from build123d import *

# Parameters (mm, degrees)
SKETCH079_W     = 100
SKETCH079_H     = 40
PAD064_DEPTH    = 5
SKETCH080_W     = 5
SKETCH080_H     = 40
PAD065_DEPTH    = 15
SKETCH081_R     = 2.7
POCKET019_DEPTH = 100.001
SKETCH082_R     = 2.7
POCKET020_DEPTH = 5
SKETCH089_W     = 90
SKETCH089_H     = 5
PAD072_DEPTH    = 15


with BuildPart() as part:
    # Sketch079 → Pad064 (new body)
    with BuildSketch(Plane.XY):
        with Locations((50, 20)):
            Rectangle(SKETCH079_W, SKETCH079_H)
    extrude(amount=PAD064_DEPTH)

    # Sketch080 (on Face6 of Pad064) → Pad065 (join)
    with BuildSketch(Plane.XY.offset(5)):
        with Locations((2.5, 20)):
            Rectangle(SKETCH080_W, SKETCH080_H)
        with Locations((97.5, 20)):
            Rectangle(SKETCH080_W, SKETCH080_H)
    extrude(amount=PAD065_DEPTH)

    # Sketch081 (on Face5 of Pad065) → Pocket019 (cut, through all)
    with BuildSketch(Plane(origin=(0, 0, 0), x_dir=(0, -1, 0), z_dir=(-1, 0, 0))):
        with Locations((-30, 10)):
            Circle(SKETCH081_R)
        with Locations((-10, 10)):
            Circle(SKETCH081_R)
    extrude(amount=-POCKET019_DEPTH, mode=Mode.SUBTRACT)

    # Sketch082 (on Face8 of Pocket019) → Pocket020 (cut)
    with BuildSketch(Plane.XY.offset(5)):
        with Locations((14, 30)):
            Circle(SKETCH082_R)
        with Locations((14, 10)):
            Circle(SKETCH082_R)
        with Locations((86, 30)):
            Circle(SKETCH082_R)
        with Locations((86, 10)):
            Circle(SKETCH082_R)
        with Locations((50, 30)):
            Circle(SKETCH082_R)
        with Locations((50, 10)):
            Circle(SKETCH082_R)
    extrude(amount=-POCKET020_DEPTH, mode=Mode.SUBTRACT)

    # Sketch089 (on Face8 of Pocket020) → Pad072 (join)
    with BuildSketch(Plane.XY.offset(5)):
        with Locations((50, 37.5)):
            Rectangle(SKETCH089_W, SKETCH089_H)
        with Locations((50, 2.5)):
            Rectangle(SKETCH089_W, SKETCH089_H)
    extrude(amount=PAD072_DEPTH)


solid = part.part
Check sheet for the modelled part. Datum: model origin and axes. Units: mm. A direction names the side the tool comes from. Give positions to 0.01 mm unless a question says otherwise; leave off trailing zeros. Order: outer loops, then holes, each group sorted by start corner. A loop starts at its lowest first (then second) coordinate and runs counter-clockwise, first axis right, second up. Notation, with made-up numbers: M -39.75,-4 L 18.25,-4 A20 cw 18.25,26 Z; hole C 54.5,48.25 d11. An arc over 180 degrees is marked long. Answer as CSV lines item,"result". Start each with the question number.
Item 1: Tool access check on faces 1 (the face through (49, 20, 0)), 2 (the face through (95, 20, 12)). Record the directions out of +Z, -Z, +X, -X, +Y, -Y that give a thin tool (end or side, any length) a straight path to the whole face; none if there is none.
Item 2: Cross-section at D-D on x = 22. Enter the section's corners in (y, z), plus the area to 3 significant figures.
Item 3: Cross-section at A-A on y = 30. Enter the section's corners in (x, z), plus the area to 3 significant figures.
Item 4: Gauge pin test, flat ends, axial feed: P1, Ø5, axis at x = 50, y = 30, coming from the -Z side; P2, Ø4, axis at x = 69, y = 29.5, coming from the +Z side. Record the tip position at first contact, or that the pin passes through.
Item 5: Cross-section at B-B on z = 3. Enter the section's corners in (x, y), plus the area to 3 significant figures.
Item 6: Mould release check, pull along X, two halves, no side actions. Record for faces 3 (the face through (97.465, 8.548, 12.277)), 4 (the face through (49, 35, 12)), 5 (the face through (0, 20, 10)), 6 (the face through (52.575, 30.811, 2.535)): +X half, -X half, draft (parallel to the pull), parting line (faces both ways), or undercut.
Item 7: Thickness scan on line 1 (Y direction, x = 50, z = 3.6); line 2 (Y direction, x = 14.5, z = 8.5); line 3 (Z direction, x = 98.05, y = 10). Record the ranges inside material, lowest first. Write a range as [from, to].
Item 8: Cross-section at C-C on x = 50. Enter the section's corners in (y, z).
Established:
1,face 1,"-Z, +X, -X, +Y, -Y"
1,face 2,"+Z"
2,outline,"M 0,0 L 40,0 L 40,20 L 35,20 L 35,5 L 5,5 L 5,20 L 0,20 Z"
2,area,"350 mm^2"
3,outline,"M 0,0 L 11.3,0 L 11.3,5 L 5,5 L 5,7.3 L 0,7.3 Z; M 0,12.7 L 5,12.7 L 5,20 L 0,20 Z; M 16.7,0 L 47.3,0 L 47.3,5 L 16.7,5 Z; M 52.7,0 L 83.3,0 L 83.3,5 L 52.7,5 Z; M 88.7,0 L 100,0 L 100,7.3 L 95,7.3 L 95,5 L 88.7,5 Z; M 95,12.7 L 100,12.7 L 100,20 L 95,20 Z"
3,area,"515 mm^2"
4,P1,"passes through"
4,P2,"stops at z = 5"
5,outline,"M 0,0 L 100,0 L 100,40 L 0,40 Z; hole C 14,10 d5.4; hole C 14,30 d5.4; hole C 50,10 d5.4; hole C 50,30 d5.4; hole C 86,10 d5.4; hole C 86,30 d5.4"
5,area,"3,860 mm^2"
6,face 3,"draft"
6,face 4,"undercut"
6,face 5,"-X half"
6,face 6,"undercut"
7,line 1,"y = [0, 7.3], [12.7, 27.3], [32.7, 40]"
7,line 2,"y = [0, 5], [35, 40]"
7,line 3,"z = [0, 7.3], [12.7, 20]"
8,outline,"M 0,0 L 7.3,0 L 7.3,5 L 5,5 L 5,20 L 0,20 Z; M 12.7,0 L 27.3,0 L 27.3,5 L 12.7,5 Z; M 32.7,0 L 40,0 L 40,20 L 35,20 L 35,5 L 32.7,5 Z"
